Input: part model. Units: mm. Frame: model coordinates. Face numbers are marked on the shaded views. A direction names the side the tool comes from. Coordinates: 2 decimals unless noted, no trailing zeros. One line per question, with ' | ' between items.
from build123d import *

# Parameters (mm, degrees)
SKETCH1_R           = 11.5
BOSS_EXTRUDE1_DEPTH = 10
FILLET1_SIZE        = 8
FILLET1_SIZE_2      = 10
SKETCH2_R           = 7
CUT_EXTRUDE1_DEPTH  = 7
SKETCH3_R           = 4.558249482
CUT_EXTRUDE2_DEPTH  = 2.5


with BuildPart() as part:
    # Sketch1 → Boss-Extrude1 (new body)
    with BuildSketch(Plane(origin=(0, 0, 0), x_dir=(1, 0, 0), z_dir=(0, 1, 0))):
        with Locations(Location((0, 0, 0), (0, 0, 270))):
            Circle(SKETCH1_R)
    extrude(amount=BOSS_EXTRUDE1_DEPTH)

    # Fillet1
    # an asymmetric fillet: 10, 8 mm, written as the material it takes off along each edge
    with BuildSketch(Plane(origin=(0, 10, 0), x_dir=(0, 0, 1), z_dir=(-1, 0, 0))) as fillet1_piece_1:
        with BuildLine():
            Bezier((11.5, -FILLET1_SIZE), (11.5, 0), (11.5 - FILLET1_SIZE_2, 0), weights=[1, 0.707106781, 1])
            Line((11.5 - FILLET1_SIZE_2, 0), (11.5, 0))
            Line((11.5, 0), (11.5, -FILLET1_SIZE))
        make_face()
    revolve(axis=Axis((0, 10, 0), (0, 1, 0)), mode=Mode.SUBTRACT)

    # Sketch2 → Cut-Extrude1 (cut)
    with BuildSketch(Plane.XZ):
        with Locations(Location((0, 0, 0), (0, 0, 270))):
            Circle(SKETCH2_R)
        Polygon((2.95, -1.703183294), (2.95, 1.703183294), (0, 3.406366588), (-2.95, 1.703183294), (-2.95, -1.703183294), (0, -3.406366588), align=None, mode=Mode.SUBTRACT)
    extrude(amount=-CUT_EXTRUDE1_DEPTH, mode=Mode.SUBTRACT)

    # Sketch3 → Cut-Extrude2 (cut)
    with BuildSketch(Plane.XZ):
        Circle(SKETCH3_R)
    extrude(amount=-CUT_EXTRUDE2_DEPTH, mode=Mode.SUBTRACT)


solid = part.part
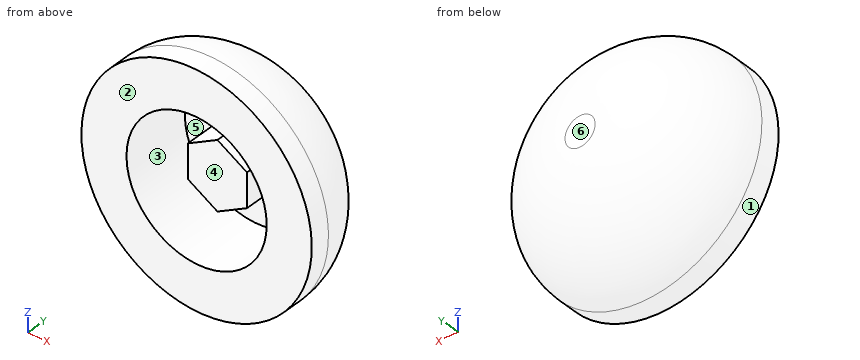
Item 1: Access query for the marked faces 5 and 6. Directions: +Z, -Z, +X, -X, +Y, -Y. A direction counts if a zero-diameter tool reaches every point of the face in a straight line with its end or side. Return the directions, or none.
Data:
face 5: -Y | face 6: +Z, -Z, +X, -X, +Y
Item 2: Section A-A on y = 5. Count the separate pieces of the cut face and the enclosed holes in it, and give its area (3 significant figures).
Data:
separate pieces: 2 | enclosed holes: 1 | area: 241 mm^2
Item 3: Ray query, line 1 (Z direction, x = -0.25, y = 4.25); line 2 (X direction, y = 3, z = 0); line 3 (X direction, y = 5, z = 0). Return the intervals inside material, ascending.
Data:
line 1: -11.09 to -7, -3.26 to 3.26, 7 to 11.09 | line 2: -11.42 to -7, -2.95 to 2.95, 7 to 11.42 | line 3: -10.77 to -7, -2.95 to 2.95, 7 to 10.77
Item 4: Contact query for flat-ended pins moving along their axis: P1, Ø2, axis at x = -6, z = -4, coming from the +Y side; P2, Ø10, axis at x = 8.5, z = 2.5, coming from the +Y side; P3, Ø5, axis at y = 5.5, z = 0, coming from the -X side. Output: stop coordinate, or through.
Data:
P1: y = 9.06 | P2: y = 9.77 | P3: x = -11.42
Item 5: Draft query along Z for the marked faces 1, 2, 3 and 4. Return one class per face: released by +Z, released by -Z, zero draft, split by the parting line, or undercut.
Data:
face 1: split by the parting line | face 2: zero draft | face 3: undercut | face 4: undercut
